Geometry check sheet. Reference: the model listing, model coordinates, mm. A direction names the side the tool comes from. Round coordinates to 2 decimals unless told otherwise and drop trailing zeros. Order: outer loops, then holes, each group sorted by start corner. A loop starts at its lowest first (then second) coordinate and runs counter-clockwise, first axis right, second up.
Autodesk Fusion 360 part; units mm, degrees
sketch "Sketch1" plane through (0, 0, 0) normal (0, 1, 0) x (1, 0, 0)
  line L0 (-0.5, 5) -> (0.5, 5)
  line L1 (0.5, -5) -> (-0.5, -5)
  arc A0 (-0.5, 4.3715) -> (-0.5, -4.3715) centre (0, 0) ccw
  arc A1 (0.5, -4.3715) -> (0.5, 4.3715) centre (0, 0) ccw
  line L2 (0.5, 5) -> (0.5, 4.3715)
  line L3 (0.5, -4.3715) -> (0.5, -5)
  line L4 (-0.5, -5) -> (-0.5, -4.3715)
  line L5 (-0.5, 4.3715) -> (-0.5, 5)
  line L6 (10.3923, -7) -> (0, 11)
  line L7 (0, 11) -> (-10.3923, -7)
  line L8 (-10.3923, -7) -> (10.3923, -7)
  point P0 (0, -1)
  point P1 (0, -1)
  dimension "d1" = 8.8
  dimension "d10" = 1
  dimension "d11" = 6
  dimension "d12" = 4.4
extrude "Extrude1" add sketch "Sketch1" along normal blind 40
extrude "Extrude2" add sketch "Sketch1" against normal blind 3 contours L0 L1 A0 A1 L2 L3 L4 L5 | L6 L7 L8
fillet "Fillet1" radius 1 8 edges at (-4.4, 40, 0) (4.4, 40, 0) (-0.5, 40, -4.6857) (0.5, 40, -4.6857) (0, 40, -5) (-0.5, 40, 4.6857) (0, 40, 5) (0.5, 40, 4.6857)
fillet "Fillet2" radius 3 3 edges at (10.3923, 18.5, 7) (-10.3923, 18.5, 7) (0, 18.5, -11)
(1) Sectioned sample at A-A, the plane y = 8. Record the cut outline in (x, z).
Returned:
outline: (-7.79, 2.5) - (-2.6, -6.5) arc R3 ccw to (2.6, -6.5) - (7.79, 2.5) arc R3 ccw to (5.2, 7) - (-5.2, 7) arc R3 ccw to start; hole (-0.5, -5) - (0.5, -5) - (0.5, -4.37) arc R4.4 ccw to (0.5, 4.37) - (0.5, 5) - (-0.5, 5) - (-0.5, 4.37) arc R4.4 ccw to (-0.5, -4.37) - close
(2) Material ranges on line 1 (Z direction, x = -3, y = 35.5); line 2 (Y direction, x = -0.25, z = -3.5); line 3 (Z direction, x = -4, y = 17), recorded low to high.
Returned:
line 1: z = -5.8 to -3.22, 3.22 to 7
line 2: y = -3 to 0
line 3: z = -4.07 to -1.83, 1.83 to 7
(3) Depth check by flat-ended pin: P1, Ø0.7, axis at y = 16, z = -5, coming from the +X side; P2, Ø6, axis at y = 31, z = -1.5, coming from the +X side; P3, Ø3, axis at x = 2, y = 22.5, coming from the -Z side. Enter the tip coordinate at first touch or a pass-through.
Returned:
P1: stops at x = 3.67
P2: stops at x = 7.22
P3: stops at z = -7.96
(4) Set-up check for faces 1 (the cylindrical face through (0.9, 39.8, -5.2)), 2 (the flat face through (0, 18, 7)): record each of +Z, -Z, +X, -X, +Y, -Y from which the full face is reachable in a straight line by a thin tool's end or side.
Returned:
face 1: +Y
face 2: +Z, +X, -X, +Y, -Y
